Build history of the part. All positions in model axes, mm. Give positions to 0.01 mm unless a question says otherwise; leave off trailing zeros. Loops run counter-clockwise (first coordinate to the right, second up) from the corner with the lowest first, then second, coordinate; pieces in that order, holes last. Notation, with made-up numbers: (72.5, -14) -> (79.5, -14) arc R22 ccw to (79.5, 4) -> close; hole circle Ø10 at (-14, 39.5). An arc over 180 degrees is marked (long way). One line per question, with ' | ' between items. Start each with the question number.
(1) Slice it at A-A, the plane z = 100. Write the cut outline in (x, y), then the cut area to 3 significant figures.
(2) Mould opens along Z. For faces 1 (the face through (97.6, 2, 101.8)), 2 (the face through (99, 4, 76)) say: pulls with the +Z half, pulls with the -Z half, needs draft (parallel to the pull), parting line crosses it, or undercut.
(3) Flat gauge pin, fed straight in: pin 1 Ø2 at (x, y) = (97.5, 1.5) entering from -Z. Where does the tip first touch, or does it go through?
(4) Drill centre lines: L1, parallel to Z at x = 94, y = 0.3; L2, parallel to Z at x = 100, y = 2.4; L3, parallel to X at y = 0.9, z = 100. Where is each one in solid material? Low to high. Write a range as from..to.
(5) Slice it at C-C, the plane x = 60. Write the cut outline in (y, z).
(6) Slice it at B-B, the plane x = 100. Write the cut outline in (y, z), then the cut area to 3 significant figures.
(7) Slice it at D-D, the plane y = 2.95. Give the number of separate pieces and of enclosed holes in the cut face, then the cut area to 3 significant figures.
```python
from build123d import *

# Parameters (mm, degrees)
SKETCH1_W           = 200
SKETCH1_H           = 200
SKETCH1_R           = 3
SKETCH1_W_2         = 15
SKETCH1_H_2         = 4
BOSS_EXTRUDE1_DEPTH = 4


with BuildPart() as part:
    # Sketch1 → Boss-Extrude1 (new body)
    with BuildSketch(Plane(origin=(0, 0, 0), x_dir=(1, 0, 0), z_dir=(0, 1, 0))):
        with Locations((100, -100)):
            Rectangle(SKETCH1_W, SKETCH1_H)
        with Locations((100, -100)):
            Circle(SKETCH1_R, mode=Mode.SUBTRACT)
        with Locations((30, -12)):
            Rectangle(SKETCH1_W_2, SKETCH1_H_2, mode=Mode.SUBTRACT)
        with Locations((65, -12)):
            Rectangle(SKETCH1_W_2, SKETCH1_H_2, mode=Mode.SUBTRACT)
        with Locations((100, -12)):
            Rectangle(SKETCH1_W_2, SKETCH1_H_2, mode=Mode.SUBTRACT)
        with Locations((135, -12)):
            Rectangle(SKETCH1_W_2, SKETCH1_H_2, mode=Mode.SUBTRACT)
        with Locations((170, -12)):
            Rectangle(SKETCH1_W_2, SKETCH1_H_2, mode=Mode.SUBTRACT)
        with Locations((170, -188)):
            Rectangle(SKETCH1_W_2, SKETCH1_H_2, mode=Mode.SUBTRACT)
        with Locations((135, -188)):
            Rectangle(SKETCH1_W_2, SKETCH1_H_2, mode=Mode.SUBTRACT)
        with Locations((100, -188)):
            Rectangle(SKETCH1_W_2, SKETCH1_H_2, mode=Mode.SUBTRACT)
        with Locations((65, -188)):
            Rectangle(SKETCH1_W_2, SKETCH1_H_2, mode=Mode.SUBTRACT)
        with Locations((30, -188)):
            Rectangle(SKETCH1_W_2, SKETCH1_H_2, mode=Mode.SUBTRACT)
    extrude(amount=BOSS_EXTRUDE1_DEPTH)


solid = part.part
```
Final values:
1) outline: (0, 0) -> (97, 0) -> (97, 4) -> (0, 4) -> close; (103, 0) -> (200, 0) -> (200, 4) -> (103, 4) -> close | area: 776 mm2
2) face 1: undercut | face 2: needs draft
3) pin 1: z = 0
4) L1: 0..10, 14..186, 190..200 | L2: 0..10, 14..97, 103..186, 190..200 | L3: 0..97, 103..200
5) outline: (0, 0) -> (4, 0) -> (4, 10) -> (0, 10) -> close; (0, 14) -> (4, 14) -> (4, 186) -> (0, 186) -> close; (0, 190) -> (4, 190) -> (4, 200) -> (0, 200) -> close
6) outline: (0, 0) -> (4, 0) -> (4, 10) -> (0, 10) -> close; (0, 14) -> (4, 14) -> (4, 97) -> (0, 97) -> close; (0, 103) -> (4, 103) -> (4, 186) -> (0, 186) -> close; (0, 190) -> (4, 190) -> (4, 200) -> (0, 200) -> close | area: 744 mm2
7) separate pieces: 1 | enclosed holes: 11 | area: 39,400 mm2
